Geometry: final body of the model. Coordinates: model frame, mm. Face numbers are marked on the shaded views. A direction names the side the tool comes from. Give positions to 0.01 mm unless a question says otherwise; leave off trailing zeros. Write each loop counter-clockwise with the first axis right and the second up, starting at its lowest first coordinate (ties: lowest second). Pieces come first, ordered by that corner, then holes.
```python
from build123d import *

# Parameters (mm, degrees)
SKETCH1_W           = 20
SKETCH1_H           = 4.75
BOSS_EXTRUDE1_DEPTH = 25
BOSS_EXTRUDE3_DEPTH = 20
SKETCH5_W           = 4.913004547
SKETCH5_H           = 2.75
CUT_EXTRUDE1_DEPTH  = 38.5807331
SKETCH9_W           = 20.464128198
SKETCH9_H           = 5.182266339
CUT_EXTRUDE3_DEPTH  = 38.5807331
SKETCH10_W          = 14.752031578
SKETCH10_H          = 2
BOSS_EXTRUDE4_DEPTH = 20
FILLET1_R           = 3
FILLET2_R           = 3
SKETCH11_W          = 20
SKETCH11_H          = 2
BOSS_EXTRUDE5_DEPTH = 10
SKETCH12_W          = 20
SKETCH12_H          = 2
BOSS_EXTRUDE6_DEPTH = 10
FILLET5_R           = 1
FILLET6_R           = 1
SKETCH13_R          = 2
CUT_EXTRUDE4_DEPTH  = 42.776882393
FILLET7_R           = 1
FILLET8_R           = 1
SKETCH14_W          = 7
SKETCH14_H          = 2
BOSS_EXTRUDE7_DEPTH = 5
SKETCH15_W          = 5
SKETCH15_H          = 9.09517733
BOSS_EXTRUDE8_DEPTH = 3
SKETCH16_W          = 20
SKETCH16_H          = 45
SKETCH16_R          = 2
BOSS_EXTRUDE9_DEPTH = 3


with BuildPart() as part:
    # Sketch1 → Boss-Extrude1 (new body)
    with BuildSketch(Plane.XY):
        with Locations((4.924657534, 1.431506849)):
            Rectangle(SKETCH1_W, SKETCH1_H)
    extrude(amount=BOSS_EXTRUDE1_DEPTH)

    # Sketch2 → Boss-Extrude3 (add)
    with BuildSketch(Plane(origin=(14.924657534, 0, 0), x_dir=(0, 0, -1), z_dir=(1, 0, 0))):
        with BuildLine():
            Line((-7.75, 3.806506849), (-4.913004547, 3.806506849))
            ThreePointArc((-4.913004547, 3.806506849), (-12.5, 19.680231206), (-20.086995453, 3.806506849))
            Line((-20.086995453, 3.806506849), (-17.25, 3.806506849))
            ThreePointArc((-17.25, 3.806506849), (-12.5, 17.680231206), (-7.75, 3.806506849))
        make_face()
    extrude(amount=-BOSS_EXTRUDE3_DEPTH)

    # Sketch5 → Cut-Extrude1 (cut, through all)
    with BuildSketch(Plane(origin=(14.924657534, 0, 0), x_dir=(0, 0, -1), z_dir=(1, 0, 0))):
        with Locations((-22.543497727, 2.431506849)):
            Rectangle(SKETCH5_W, SKETCH5_H)
        with Locations((-2.456502273, 2.431506849)):
            Rectangle(SKETCH5_W, SKETCH5_H)
    extrude(amount=-CUT_EXTRUDE1_DEPTH, mode=Mode.SUBTRACT)

    # Sketch9 → Cut-Extrude3 (cut, through all)
    with BuildSketch(Plane(origin=(14.924657534, 0, 0), x_dir=(0, 0, -1), z_dir=(1, 0, 0))):
        with Locations((-12.097906115, 18.897640018)):
            Rectangle(SKETCH9_W, SKETCH9_H)
    extrude(amount=-CUT_EXTRUDE3_DEPTH, mode=Mode.SUBTRACT)

    # Sketch10 → Boss-Extrude4 (add)
    with BuildSketch(Plane(origin=(14.924657534, 0, 0), x_dir=(0, 0, -1), z_dir=(1, 0, 0))):
        with Locations((-12.5, 17.306506849)):
            Rectangle(SKETCH10_W, SKETCH10_H)
    extrude(amount=-BOSS_EXTRUDE4_DEPTH)

    # Fillet1
    # the kernel refuses this fillet: 3 mm, written as the material it takes off along each edge
    with BuildSketch(Plane(origin=(21.995725346, 18.306506849, 5.123984211), x_dir=(0, -1, 0), z_dir=(-1, 0, 0))) as fillet1_piece_1:
        with BuildLine():
            CenterArc((3, 2.828427125), FILLET1_R, 180, 70.528779366)
            Line((0, 2.828427125), (-0.06, 2.828427125))
            Line((-0.06, 2.828427125), (-0.06, 0))
            Line((-0.06, 0), (0, -0.06))
            ThreePointArc((0, -0.06), (1, -0.06), (1.98, -0.056568542))
            Line((1.98, -0.056568542), (2, 0))
        make_face()
    extrude(amount=34.142135624, mode=Mode.SUBTRACT)

    # Fillet2
    # the kernel refuses this fillet: 3 mm, written as the material it takes off along each edge
    with BuildSketch(Plane(origin=(21.995725346, 18.306506849, 19.876015789), x_dir=(0, -1, 0), z_dir=(-1, 0, 0))) as fillet2_piece_1:
        with BuildLine():
            CenterArc((3, -2.828427125), FILLET2_R, 109.471220634, 70.528779366)
            Line((0, -2.828427125), (-0.06, -2.828427125))
            Line((-0.06, -2.828427125), (-0.06, 0))
            Line((-0.06, 0), (0, 0.06))
            ThreePointArc((0, 0.06), (1, 0.06), (1.98, 0.056568542))
            Line((1.98, 0.056568542), (2, 0))
        make_face()
    extrude(amount=34.142135624, mode=Mode.SUBTRACT)

    # Sketch11 → Boss-Extrude5 (add)
    with BuildSketch(Plane(origin=(0, 0, 0), x_dir=(-1, 0, 0), z_dir=(0, 0, -1))):
        with Locations((-4.924657534, 0.056506849)):
            Rectangle(SKETCH11_W, SKETCH11_H)
    extrude(amount=BOSS_EXTRUDE5_DEPTH)

    # Sketch12 → Boss-Extrude6 (add)
    with BuildSketch(Plane.XY.offset(25)):
        with Locations((4.924657534, 0.056506849)):
            Rectangle(SKETCH12_W, SKETCH12_H)
    extrude(amount=BOSS_EXTRUDE6_DEPTH)

    # Fillet5
    fillet5_edges = [part.edges().sort_by_distance(p)[0] for p in [
        (4.924657534, 1.056506849, 35),
    ]]
    fillet(fillet5_edges, radius=FILLET5_R)

    # Fillet6
    fillet6_edges = [part.edges().sort_by_distance(p)[0] for p in [
        (4.924657534, 1.056506849, -10),
    ]]
    fillet(fillet6_edges, radius=FILLET6_R)

    # Sketch13 → Cut-Extrude4 (cut, through all)
    with BuildSketch(Plane(origin=(0, 1.056506849, 0), x_dir=(1, 0, 0), z_dir=(0, 1, 0))):
        with Locations(Location((-2.075342466, -28, 0), (0, 0, 270))):
            Circle(SKETCH13_R)
        with Locations(Location((11.924657534, -28, 0), (0, 0, 270))):
            Circle(SKETCH13_R)
        with Locations(Location((11.924657534, 3, 0), (0, 0, 270))):
            Circle(SKETCH13_R)
        with Locations(Location((-2.075342466, 3, 0), (0, 0, 270))):
            Circle(SKETCH13_R)
    extrude(amount=-CUT_EXTRUDE4_DEPTH, mode=Mode.SUBTRACT)

    # Fillet7
    fillet7_edges = [part.edges().sort_by_distance(p)[0] for p in [
        (4.924657534, 1.056506849, 20.086995453),
    ]]
    fillet(fillet7_edges, radius=FILLET7_R)

    # Fillet8
    fillet8_edges = [part.edges().sort_by_distance(p)[0] for p in [
        (4.924657534, 1.056506849, 4.913004547),
    ]]
    fillet(fillet8_edges, radius=FILLET8_R)



with BuildPart() as body_2:
    # Sketch14 → Boss-Extrude7 (new body)
    with BuildSketch(Plane.ZY.offset(5.075342466)):
        with Locations((12.767411335, 17.306506849)):
            Rectangle(SKETCH14_W, SKETCH14_H)
    extrude(amount=BOSS_EXTRUDE7_DEPTH)


with BuildPart() as part_1:
    add(part.part)

    add(body_2.part)  # Boss-Extrude8 merges body 2
    # Sketch15 → Boss-Extrude8 (add)
    with BuildSketch(Plane.XZ.offset(-18.306506849)):
        with Locations((-7.575342466, 12.5)):
            Rectangle(SKETCH15_W, SKETCH15_H)
    extrude(amount=BOSS_EXTRUDE8_DEPTH)

    # Sketch16 → Boss-Extrude9 (add)
    with BuildSketch(Plane.XZ.offset(0.943493151)):
        with Locations((4.924657534, 12.5)):
            Rectangle(SKETCH16_W, SKETCH16_H)
        with Locations(Location((11.924657534, -3, 0), (0, 0, 90))):
            Circle(SKETCH16_R, mode=Mode.SUBTRACT)
        with Locations(Location((11.924657534, 28, 0), (0, 0, 90))):
            Circle(SKETCH16_R, mode=Mode.SUBTRACT)
        with Locations(Location((-2.075342466, 28, 0), (0, 0, 90))):
            Circle(SKETCH16_R, mode=Mode.SUBTRACT)
        with Locations(Location((-2.075342466, -3, 0), (0, 0, 90))):
            Circle(SKETCH16_R, mode=Mode.SUBTRACT)
    extrude(amount=BOSS_EXTRUDE9_DEPTH)


solid = part_1.part
```
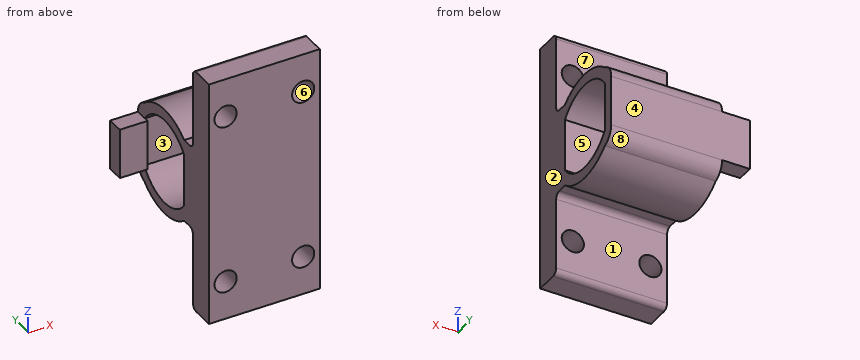
Item 1: Line query: L1, parallel to X at y = 0.05, z = 28; L2, parallel to Y at x = 1, z = 9.5; L3, parallel to Z at x = -1.75, y = 9.75. Output: solid intervals per line, ascending.
Found:
L1: x = -5.08 to -4.08, -0.08 to 9.92, 13.92 to 14.92
L2: y = -3.94 to 3.81, 16.31 to 18.31
L3: z = 2.75 to 4.75, 20.25 to 22.25
Item 2: Section B-B, the plane z = 28. Return the cut outline in (x, y), plus the area to 3 significant figures.
Found:
outline: (-5.08, -3.94) - (-4.08, -3.94) - (-4.08, 1.06) - (-5.08, 1.06) - close; (-0.08, -3.94) - (9.92, -3.94) - (9.92, 1.06) - (-0.08, 1.06) - close; (13.92, -3.94) - (14.92, -3.94) - (14.92, 1.06) - (13.92, 1.06) - close
area: 60.0 mm2
Item 3: Pin query (flat end, axial travel): pin 1 Ø4.5 at (x, z) = (-2.08, -3) entering from +Y; pin 2 Ø8 at (x, y) = (2.5, 8) entering from +Z; pin 3 Ø2 at (x, y) = (7, 16) entering from +Z. Return the tip coordinate at first contact, or that it passes through.
Found:
pin 1: stops at y = 1.06
pin 2: stops at z = 22.25
pin 3: stops at z = 20.83
Item 4: Section D-D, the plane x = 10.5. Return the cut outline in (y, z).
Found:
outline: (-3.94, -10) - (0.06, -10) arc R1 ccw to (1.06, -9) - (1.06, -4.4) - (-3.94, -4.4) - close; (-3.94, -1.6) - (1.06, -1.6) - (1.06, 3.91) arc R1 cw to (2.06, 4.91) - (3.81, 4.91) arc R9.75 ccw to (16.31, 5.12) arc R3 ccw to (18.31, 7.95) - (18.31, 17.05) arc R3 ccw to (16.31, 19.88) arc R9.75 ccw to (3.81, 20.09) - (2.06, 20.09) arc R1 cw to (1.06, 21.09) - (1.06, 26.6) - (-3.94, 26.6) - close; (-3.94, 29.4) - (1.06, 29.4) - (1.06, 34) arc R1 ccw to (0.06, 35) - (-3.94, 35) - close; hole (3.81, 7.75) arc R7.75 ccw to (16.31, 8.09) - (16.31, 16.91) arc R7.75 ccw to (3.81, 17.25) - close
Item 5: Section C-C, the plane z = 15. Return the cut outline in (x, y), plus the area to 3 significant figures.
Found:
outline: (-10.08, 15.31) - (-5.08, 15.31) - (-5.08, 16.31) - (14.92, 16.31) - (14.92, 18.31) - (-10.08, 18.31) - close; (-5.08, -3.94) - (14.92, -3.94) - (14.92, 3.81) - (-5.08, 3.81) - close
area: 210 mm2
Item 6: Pull-direction query (Z, two-part tool) for the marked faces 6, 7 and 8; classes: +Z half, -Z half, draft (parallel to the pull), parting line (faces both ways), or undercut.
Found:
face 6: undercut
face 7: draft
face 8: -Z half
Item 7: Reachability of the marked faces 1, 2, 3, 4 and 5 from +Z, -Z, +X, -X, +Y, -Y: full face, straight path, thin tool, end or side. Return the list, or none.
Found:
face 1: -Z, +X, -X
face 2: +Z, -Z, +X, +Y, -Y
face 3: +X
face 4: +Z, -Z, +X, -X, +Y
face 5: +X, -X
Item 8: Section A-A, the plane x = 7.75. Return the cut outline in (y, z), plus the area to 3 significant figures.
Found:
outline: (-3.94, -10) - (0.06, -10) arc R1 ccw to (1.06, -9) - (1.06, 3.91) arc R1 cw to (2.06, 4.91) - (3.81, 4.91) arc R9.75 ccw to (16.31, 5.12) arc R3 ccw to (18.31, 7.95) - (18.31, 17.05) arc R3 ccw to (16.31, 19.88) arc R9.75 ccw to (3.81, 20.09) - (2.06, 20.09) arc R1 cw to (1.06, 21.09) - (1.06, 34) arc R1 ccw to (0.06, 35) - (-3.94, 35) - close; hole (3.81, 7.75) arc R7.75 ccw to (16.31, 8.09) - (16.31, 16.91) arc R7.75 ccw to (3.81, 17.25) - close
area: 349 mm2
